Job drawing, mm, ordinate dimensions from the low corner. One solid piece. A direction names the side the tool comes from. Give positions to 0.01 mm unless a question says otherwise; leave off trailing zeros. Order: outer loops, then holes, each group sorted by start corner. A loop starts at its lowest first (then second) coordinate and runs counter-clockwise, first axis right, second up.
Item 1: Flat gauge pins, fed straight in: P1, Ø3.5, axis at x = 45, z = 5, coming from the +Y side; P2, Ø0.8, axis at y = 3.5, z = 9.5, coming from the +X side; P3, Ø0.8, axis at y = 3.5, z = 12, coming from the -X side. Where does each tip first touch, or does it go through?
Item 2: Which spindle directions (+Z, -Z, +X, -X, +Y, -Y) get a long thin tool onto all of the face, cutting with end or side? Do the marked faces 1, 2, 3, 4 and 5. Say none if no direction does.
Item 3: Band-saw the part on D-D on z = 7.75. Give the cut face in (x, y).
Item 4: Two-plate mould, pull along X, no slides. Class the marked faces 6 and 7: released by +X, released by -X, zero draft, split by the parting line, or undercut.
Item 5: Band-saw the part on B-B on x = 5. Give the cut face in (y, z), plus the area to 3 significant figures.
Item 6: Band-saw the part on C-C on z = 15. Give the cut face in (x, y).
Item 7: Wall check: L1, parallel to Z at x = 5, y = 2.65; L2, parallel to X at y = 1.3, z = 15; L3, parallel to Z at x = 14, y = 3.05. Give the ranges that are in metal, low to high.
Item 8: Band-saw the part on A-A on y = 2.5. Count the separate pieces of the cut face and the enclosed holes in it, plus the area to 3 significant figures.
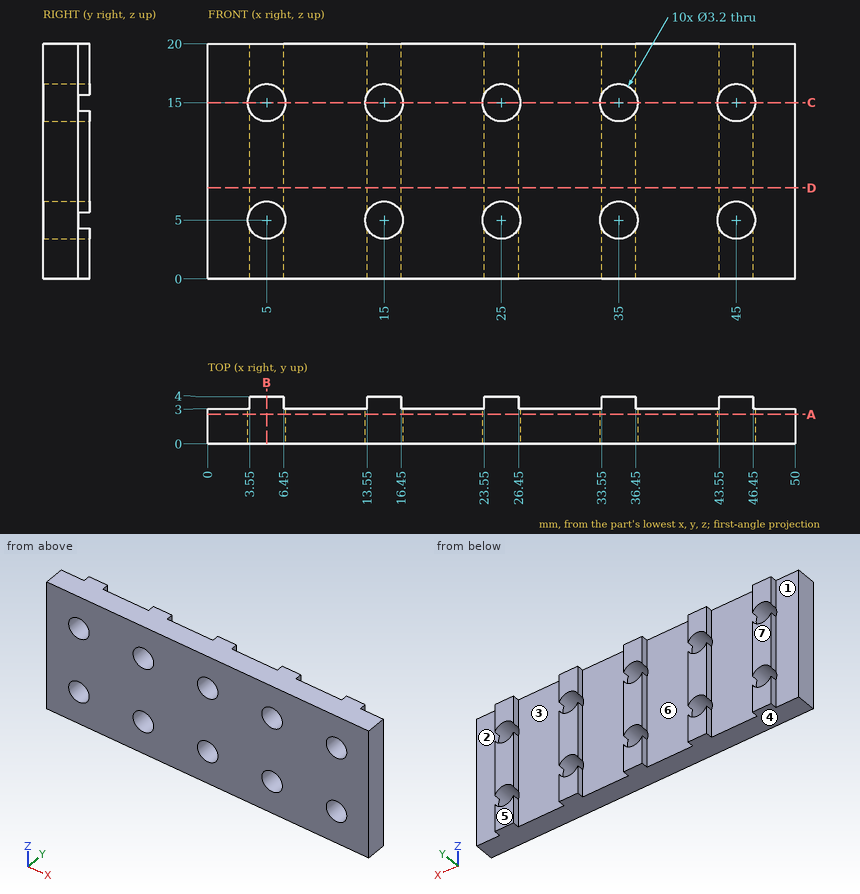
The answers:
1. P1: stops at y = 4
1. P2: stops at x = 46.45
1. P3: stops at x = 3.55
2. face 1: +Z, -Z, -X, +Y
2. face 2: +Z, -Z, +X, +Y
2. face 3: +Z, -Z, +Y
2. face 4: -Z, +X, -X, +Y, -Y
2. face 5: +Z, -Z, +X, -X, +Y
3. outline: (0, 0) - (50, 0) - (50, 3) - (46.45, 3) - (46.45, 4) - (43.55, 4) - (43.55, 3) - (36.45, 3) - (36.45, 4) - (33.55, 4) - (33.55, 3) - (26.45, 3) - (26.45, 4) - (23.55, 4) - (23.55, 3) - (16.45, 3) - (16.45, 4) - (13.55, 4) - (13.55, 3) - (6.45, 3) - (6.45, 4) - (3.55, 4) - (3.55, 3) - (0, 3) - close
4. face 6: undercut
4. face 7: zero draft
5. outline: (0, 0) - (4, 0) - (4, 3.4) - (0, 3.4) - close; (0, 6.6) - (4, 6.6) - (4, 13.4) - (0, 13.4) - close; (0, 16.6) - (4, 16.6) - (4, 20) - (0, 20) - close
5. area: 54.4 mm2
6. outline: (0, 0) - (3.4, 0) - (3.4, 3) - (0, 3) - close; (6.6, 0) - (13.4, 0) - (13.4, 3) - (6.6, 3) - close; (16.6, 0) - (23.4, 0) - (23.4, 3) - (16.6, 3) - close; (26.6, 0) - (33.4, 0) - (33.4, 3) - (26.6, 3) - close; (36.6, 0) - (43.4, 0) - (43.4, 3) - (36.6, 3) - close; (46.6, 0) - (50, 0) - (50, 3) - (46.6, 3) - close
7. L1: z = 0 to 3.4, 6.6 to 13.4, 16.6 to 20
7. L2: x = 0 to 3.4, 6.6 to 13.4, 16.6 to 23.4, 26.6 to 33.4, 36.6 to 43.4, 46.6 to 50
7. L3: z = 0 to 3.75, 6.25 to 13.75, 16.25 to 20
8. separate pieces: 1
8. enclosed holes: 10
8. area: 920 mm2
